Design review of the part built by this model. Coordinates are the model's own, in mm. Face numbers are marked on the shaded views. A direction names the side the tool comes from. Give positions to 0.01 mm unless a question says otherwise; leave off trailing zeros. Write each loop counter-clockwise with the first axis right and the second up, starting at its lowest first coordinate (ties: lowest second). Pieces come first, ordered by that corner, then holes. Notation, with made-up numbers: (53.5, 75.25) -> (63.5, 75.25) arc R4 cw to (63.5, 80.25) -> close; hole circle Ø9 at (-4.5, 84.5). An arc over 180 degrees is marked (long way). Return JSON: item names as keys, results as strings. Group by question number.
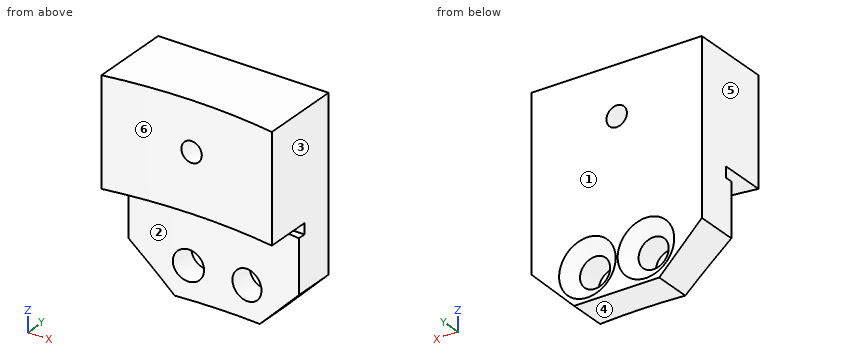
from build123d import *

# Parameters (mm, degrees)
SKETCH1_W                                         = 25.4
SKETCH1_H                                         = 31.75
BOSS_EXTRUDE1_DEPTH                               = 6.35
CUT_EXTRUDE1_DEPTH                                = 35.780382402
BOSS_EXTRUDE2_DEPTH                               = 15.875
SKETCH4_W                                         = 1.5875
SKETCH4_H                                         = 1.190625
CUT_EXTRUDE2_DEPTH                                = 31.618591166
CHAMFER1_SIZE                                     = 6.35
SKETCH5_R                                         = 1.524
CUT_EXTRUDE3_DEPTH                                = 24.692140063
CSK_FOR_8_FLAT_HEAD_MACHINE_SCREW_100_D           = 4.4958
CSK_FOR_8_FLAT_HEAD_MACHINE_SCREW_100_CSINK_D     = 8.4328
CSK_FOR_8_FLAT_HEAD_MACHINE_SCREW_100_CSINK_ANGLE = 100


with BuildPart() as part:
    # Sketch1 → Boss-Extrude1 (new body)
    with BuildSketch(Plane(origin=(0, 0, 0), x_dir=(1, 0, 0), z_dir=(0, 1, 0))):
        Rectangle(SKETCH1_W, SKETCH1_H)
    extrude(amount=BOSS_EXTRUDE1_DEPTH)

    # Sketch2 → Cut-Extrude1 (cut, through all)
    with BuildSketch(Plane.XY.offset(15.875)):
        with BuildLine():
            Line((-12.7, 0), (12.7, 0))
            ThreePointArc((12.7, 0), (0, 0.990173613), (-12.7, 0))
        make_face()
    extrude(amount=-CUT_EXTRUDE1_DEPTH, mode=Mode.SUBTRACT)

    # Sketch3 → Boss-Extrude2 (add)
    with BuildSketch(Plane.XY.offset(15.875)):
        with BuildLine():
            Line((-12.7, 6.35), (12.7, 6.35))
            Line((12.7, 6.35), (12.7, -5.816013142))
            ThreePointArc((12.7, -5.816013142), (0, -4.750226387), (-12.7, -5.816013142))
            Line((-12.7, -5.816013142), (-12.7, 6.35))
        make_face()
    extrude(amount=-BOSS_EXTRUDE2_DEPTH)

    # Sketch4 → Cut-Extrude2 (cut, through all)
    with BuildSketch(Plane.ZY.offset(12.7)):
        with Locations((-0.79375, 0.5953125)):
            Rectangle(SKETCH4_W, SKETCH4_H)
    extrude(amount=-CUT_EXTRUDE2_DEPTH, mode=Mode.SUBTRACT)

    # Chamfer1
    chamfer1_edges = [part.edges().sort_by_distance(p)[0] for p in [
        (-12.7, 3.175, -15.875),
        (12.7, 3.175, -15.875),
    ]]
    chamfer(chamfer1_edges, length=CHAMFER1_SIZE)

    # Sketch5 → Cut-Extrude3 (cut, through all)
    with BuildSketch(Plane(origin=(0, 6.35, 0), x_dir=(1, 0, 0), z_dir=(0, 1, 0))):
        with Locations(Location((0, -8.636, 0), (0, 0, 270))):
            Circle(SKETCH5_R)
    extrude(amount=-CUT_EXTRUDE3_DEPTH, mode=Mode.SUBTRACT)

    # CSK for #8 Flat Head Machine Screw (100)1 (through all)
    with Locations(Plane(origin=(0, 6.35, 0), x_dir=(1, 0, 0), z_dir=(0, 1, 0))):
        with Locations((-4.365625, 11.1125), (4.365625, 11.1125)):
            CounterSinkHole(CSK_FOR_8_FLAT_HEAD_MACHINE_SCREW_100_D / 2, CSK_FOR_8_FLAT_HEAD_MACHINE_SCREW_100_CSINK_D / 2, counter_sink_angle=CSK_FOR_8_FLAT_HEAD_MACHINE_SCREW_100_CSINK_ANGLE)


solid = part.part
Q1. Take a section at D-D, the plane z = -5. Give the boundary of the cut face in (x, y), plus the area to 3 significant figures.
Q2. Take a section at C-C, the plane y = 5.75. Count the separate pieces of the cut face and the enclosed holes in it, plus the area to 3 significant figures.
Q3. Take a section at B-B, the plane y = -4.25. Give the boundary of the cut face in (x, z) (3 decimals).
Q4. Insertion check: pin 1 (2 mm diameter, centred on x = 1, y = -2, fed in from -Z); pin 2 (2.5 mm diameter, centred on x = -4.37, z = -11.11, fed in from +Y); pin 3 (1.7 mm diameter, centred on x = -2.5, z = -1, fed in from -Y); pin 4 (6 mm diameter, centred on x = 4.37, z = -11.11, fed in from +Y). Each pin has a flat end and moves straight along its axis. Give the tip position at first contact, or say it passes through.
Q5. For L1, parallel to Z at x = 0, y = -2.25 (3 decimals); L2, parallel to X at y = -0.75, z = 8.5; L3, parallel to Z at x = 1.75, y = -3 (3 decimals), list the stretches that pass through material, from the lowest coordinate up. Write a range as from..to.
Q6. Mouldability with a two-part tool opening along X and no side actions: class the marked faces 3, 4, 5 and 6 as +X half, -X half, draft (parallel to the pull), parting line (faces both ways), or undercut.
Q7. Tool access review of the marked faces 1 and 2: name each direction out of +Z, -Z, +X, -X, +Y, -Y from which nothing blocks a thin tool from reaching the whole face with its end or side.
Q8. Take a section at A-A, the plane z = 8.5. Give the boundary of the cut face in (x, y), plus the area to 3 significant figures.
Final values:
{
 "1": {"outline": "(-12.7, 0) arc R81.94 cw to (12.7, 0) -> (12.7, 6.35) -> (-12.7, 6.35) -> close", "area": "145 mm²"},
 "2": {"separate pieces": "1", "enclosed holes": "3", "area": "682 mm²"},
 "3": {"outline": "(-12.7, 0) -> (12.7, 0) -> (12.7, 15.875) -> (-12.7, 15.875) -> close; hole circle Ø3.048 at (0, 8.636)"},
 "4": {"pin 1": "stops at z = 0", "pin 2": "passes through", "pin 3": "stops at y = 0.93", "pin 4": "stops at y = 5.33"},
 "5": {"L1": "z = 0..7.112, 10.16..15.875", "L2": "x = -12.7..-1.52, 1.52..12.7", "L3": "z = 0..15.875"},
 "6": {"face 3": "+X half", "face 4": "draft", "face 5": "-X half", "face 6": "undercut"},
 "7": {"face 1": "+Z, -Z, +X, -X, +Y", "face 2": "-Z, -Y"},
 "8": {"outline": "(-12.7, -5.82) arc R76.2 cw to (-1.52, -4.77) -> (-1.52, 6.35) -> (-12.7, 6.35) -> close; (1.52, -4.77) arc R76.2 cw to (12.7, -5.82) -> (12.7, 6.35) -> (1.52, 6.35) -> close", "area": "257 mm²"}
}
